Geometry: see drawing. Coordinates: mm, zero at the bounding-box minimum. Give positions to 0.01 mm unless a question says otherwise; leave off trailing zeros. Loops run counter-clockwise (first coordinate to the right, second up) from the corner with the lowest first, then second, coordinate; pieces in that order, holes last. Notation, with made-up numbers: (44.5, -9) -> (57.5, -9) arc R29 ccw to (57.5, 20) -> close; hole circle Ø5 at (36.25, 12.5). An arc over 180 degrees is marked (long way). Return JSON: item names as keys, results as strings. Group by question number.
(1) Cut plane D-D on y = 2.25. Return loops of the section in (x, z).
(2) Draft query along Z for the marked faces 1, 2 and 3. Return one class per face: released by +Z, released by -Z, zero draft, split by the parting line, or undercut.
(3) Cut plane B-B on x = 35. Return loops of the section in (y, z), then the cut area to 3 significant figures.
(4) Pin query (flat end, axial travel): pin 1 (1 mm diameter, centred on x = 41, y = 12.5, fed in from -Z); pin 2 (4 mm diameter, centred on x = 39, z = 23, fed in from -Y); pin 3 (8 mm diameter, centred on x = 32, z = 39.5, fed in from +Y); pin 4 (2 mm diameter, centred on x = 60, y = 2.5, fed in from +Z). Return the tip coordinate at first contact, or that it passes through.
(5) Cut plane C-C on y = 13.75. Return loops of the section in (x, z).
(6) Ray query, line 1 (X direction, y = 11.5, z = 35); line 2 (Y direction, x = 34.5, z = 5). Return the intervals inside material, ascending. Write a range as from..to.
(7) Cut plane A-A on z = 35. Return loops of the section in (x, y), then the cut area to 3 significant figures.
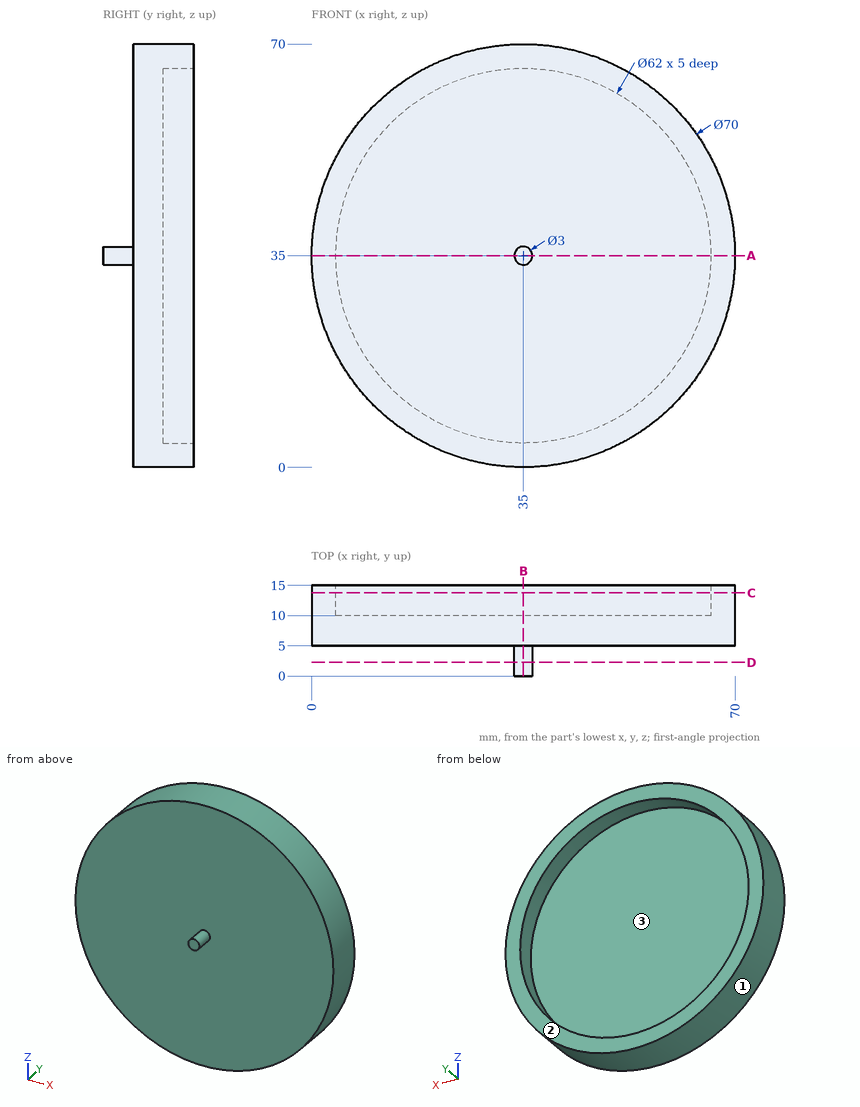
Answers:
{
 "1": {"outline": "circle Ø3 at (35, 35)"},
 "2": {"face 1": "split by the parting line", "face 2": "zero draft", "face 3": "undercut"},
 "3": {"outline": "(0, 33.5) -> (5, 33.5) -> (5, 0) -> (15, 0) -> (15, 4) -> (10, 4) -> (10, 66) -> (15, 66) -> (15, 70) -> (5, 70) -> (5, 36.5) -> (0, 36.5) -> close", "area": "405 mm²"},
 "4": {"pin 1": "z = 0.43", "pin 2": "y = 5", "pin 3": "y = 10", "pin 4": "through"},
 "5": {"outline": "circle Ø70 at (35, 35); hole circle Ø62 at (35, 35)"},
 "6": {"line 1": "0..4, 66..70", "line 2": "5..10"},
 "7": {"outline": "(0, 5) -> (33.5, 5) -> (33.5, 0) -> (36.5, 0) -> (36.5, 5) -> (70, 5) -> (70, 15) -> (66, 15) -> (66, 10) -> (4, 10) -> (4, 15) -> (0, 15) -> close", "area": "405 mm²"}
}
